Check sheet for the modelled part. Datum: model origin and axes. Units: mm. Face numbers are marked on the shaded views. A direction names the side the tool comes from. Coordinates: 2 decimals unless noted, no trailing zeros. Order: outer loops, then holes, each group sorted by start corner. A loop starts at its lowest first (then second) coordinate and runs counter-clockwise, first axis right, second up.
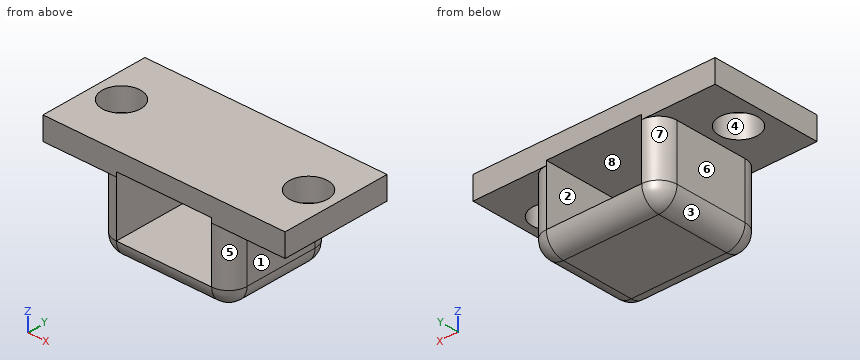
Autodesk Inventor part; units mm, degrees
ref_plane "YZ Plane" through (0, 0, 0) normal (1, 0, 0) x (0, 1, 0)
ref_plane "XZ Plane" through (0, 0, 0) normal (0, 1, 0) x (-1, 0, 0)
ref_plane "XY Plane" through (0, 0, 0) normal (0, 0, 1) x (1, 0, 0)
sketch "Sketch1" plane through (0, 0, 0) normal (0, 1, 0) x (-1, 0, 0)
  line L0 (5.2, 3.25) -> (-5.2, 3.25)
  line L1 (-5.2, 3.25) -> (-5.2, -3.25)
  line L2 (-5.2, -3.25) -> (5.2, -3.25)
  line L3 (5.2, -3.25) -> (5.2, 3.25)
  line L4 (0, -3.25) -> (0, 3.25) construction
  line L5 (5.2, 0) -> (-5.2, 0) construction
  line L6 (7.2, -5.25) -> (-7.2, -5.25)
  line L7 (-7.2, -5.25) -> (-7.2, 5.25)
  line L8 (-7.2, 5.25) -> (7.2, 5.25)
  line L9 (7.2, 5.25) -> (7.2, -5.25)
  line L10 (-13.2, 2.75) -> (-7.2, 2.75)
  line L11 (-7.2, 2.75) -> (-7.2, 5.25)
  line L12 (-7.2, 5.25) -> (-13.2, 5.25)
  line L13 (-13.2, 5.25) -> (-13.2, 2.75)
  line L14 (7.2, 2.75) -> (13.2, 2.75)
  line L15 (13.2, 2.75) -> (13.2, 5.25)
  line L16 (13.2, 5.25) -> (7.2, 5.25)
  line L17 (7.2, 5.25) -> (7.2, 2.75)
  point P0 (0, 0)
  dimension "d0" = 10.4
  dimension "d1" = 6.5
  dimension "d4" = 2
  dimension "d5" = 2
  dimension "d6" = 2
  dimension "d7" = 2
  dimension "d8" = 2.5
  dimension "d9" = 2.5
  dimension "d10" = 6
  dimension "d11" = 6
extrude "Extrusion2" add sketch "Sketch1" along normal blind 12
sketch "Sketch2" plane through (13.2, 0, 2.75) normal (0, 0, -1) x (-1, 0, 0)
  line L0 (26.4, 0) -> (20.4, 0) construction
  line L1 (20.4, 0) -> (20.4, 12) construction
  line L2 (20.4, 12) -> (26.4, 12) construction
  line L3 (26.4, 12) -> (26.4, 0) construction
  line L4 (20.4, 0) -> (26.4, 0) construction
  line L5 (26.4, 0) -> (26.4, 12) construction
  line L6 (20.4, 0) -> (20.4, 12) construction
  line L7 (20.4, 12) -> (26.4, 12) construction
  line L8 (23.4, 0) -> (23.4, 12) construction
  line L9 (26.4, 6) -> (20.4, 6) construction
  circle A0 centre (15.4635, 5.7038) radius 3.0285
  circle A1 centre (23.4, 6) radius 2.1
  line L10 (13.2, -1.4538) -> (13.2, 18.2002) construction
  circle A2 centre (3, 6) radius 2.1
  point P0 (13.2, 0)
  point P1 (23.4, 6)
  dimension "d15" = 4.2
extrude "Extrusion3" cut sketch "Sketch2" against normal up to surface (2.5 mm away) contours A1 | A2
fillet "Fillet1" radius 2 4 edges at (7.2, 6, -5.25) (-7.2, 6, -5.25) (0, 12, -5.25) (0, 0, -5.25)
fillet "Fillet2" radius 2 8 edges at (-6.6142, 11.4142, -4.6642) (-7.2, 12, -0.25) (6.6142, 11.4142, -4.6642) (7.2, 12, -0.2501) (6.6142, 0.5858, -4.6642) (7.2, 0, -0.2501) (-6.6142, 0.5858, -4.6642) (-7.2, 0, -0.25)
equation "\"d5\" = d4"
equation "\"d6\" = d4"
equation "\"d7\" = d4"
equation "\"d9\" = d8"
equation "\"d10\" = d11"
properties part number "USBholder version 1"
(1) Cross-section at A-A (z = 0.75). Enter the section's corners in (x, y).
Filled in:
outline: (-7.2, 2) arc R2 ccw to (-5.2, 0) - (-5.2, 12) arc R2 ccw to (-7.2, 10) - close; (5.2, 0) arc R2 ccw to (7.2, 2) - (7.2, 10) arc R2 ccw to (5.2, 12) - close
(2) Thickness scan on probe 1 along X at (y, z) = (7.25, -2); probe 2 along Y at (x, z) = (-10.2, 3.8); probe 3 along Z at (x, y) = (-1.75, 6.25). Record the ranges inside material, lowest first.
Filled in:
probe 1: x = -7.2 to -5.2, 5.2 to 7.2
probe 2: y = 0 to 3.9, 8.1 to 12
probe 3: z = -5.25 to -3.25, 3.25 to 5.25
(3) Tool access check on the marked faces 4, 5, 6, 7 and 8. Record the directions out of +Z, -Z, +X, -X, +Y, -Y that give a thin tool (end or side, any length) a straight path to the whole face; none if there is none.
Filled in:
face 4: +Z, -Z
face 5: -Z, +X, -Y
face 6: -Z, -X, +Y, -Y
face 7: -Z, -X, +Y
face 8: +Y, -Y
(4) Go/stop test with flat-tipped pins: P1, Ø5, axis at x = -3.5, z = -0.5, coming from the -Y side; P2, Ø2, axis at y = 7, z = -1.5, coming from the +X side; P3, Ø1, axis at x = -6.5, y = 8, coming from the -Z side; P4, Ø3, axis at y = 6, z = -1, coming from the -X side. Record where each tip stops, or that it passes through.
Filled in:
P1: stops at y = 0
P2: stops at x = 7.2
P3: stops at z = -5.08
P4: stops at x = -7.2
(5) Release check for a two-part mould opening along Z. For the marked faces 1, 2 and 3 record: +Z half, -Z half, draft (parallel to the pull), parting line (faces both ways), or undercut.
Filled in:
face 1: draft
face 2: undercut
face 3: -Z half
(6) Cross-section at D-D (z = 4.25). Enter the section's corners in (x, y), and give its area (3 significant figures).
Filled in:
outline: (-13.2, 0) - (13.2, 0) - (13.2, 12) - (-13.2, 12) - close; hole circle Ø4.2 at (-10.2, 6); hole circle Ø4.2 at (10.2, 6)
area: 289 mm2
(7) Cross-section at B-B (y = 6). Enter the section's corners in (x, z).
Filled in:
outline: (-13.2, 2.75) - (-12.3, 2.75) - (-12.3, 5.25) - (-13.2, 5.25) - close; (-8.1, 2.75) - (-7.2, 2.75) - (-7.2, -3.25) arc R2 ccw to (-5.2, -5.25) - (5.2, -5.25) arc R2 ccw to (7.2, -3.25) - (7.2, 2.75) - (8.1, 2.75) - (8.1, 5.25) - (-8.1, 5.25) - close; (12.3, 2.75) - (13.2, 2.75) - (13.2, 5.25) - (12.3, 5.25) - close; hole (-5.2, -3.25) - (5.2, -3.25) - (5.2, 3.25) - (-5.2, 3.25) - close
